```python
from build123d import *

# Parameters (mm, degrees)
BOSS_EXTRUDE1_DEPTH         = 4.7625
F_6_CLEARANCE_HOLE1_D       = 4.3053
F_3_4_0_75_DIAMETER_HOLE1_D = 19.05


with BuildPart() as part:
    # Sketch1 → Boss-Extrude1 (new body)
    with BuildSketch(Plane.XY):
        with BuildLine():
            Line((-159.14246691, -0.79375), (-164.887315329, -10.744119343))
            ThreePointArc((-164.887315329, -10.744119343), (-165.045907249, -11.126994109), (-165.1, -11.537869343))
            Line((-165.1, -11.537869343), (-165.1, -23.8125))
            ThreePointArc((-165.1, -23.8125), (-164.635032015, -24.935032015), (-163.5125, -25.4))
            Line((-163.5125, -25.4), (-1.5875, -25.4))
            ThreePointArc((-1.5875, -25.4), (-0.464967985, -24.935032015), (0, -23.8125))
            Line((0, -23.8125), (0, -1.5875))
            ThreePointArc((0, -1.5875), (-0.464967985, -0.464967985), (-1.5875, 0))
            Line((-1.5875, 0), (-157.767651581, 0))
            ThreePointArc((-157.767651581, 0), (-158.561401581, -0.212684671), (-159.14246691, -0.79375))
        make_face()
    extrude(amount=BOSS_EXTRUDE1_DEPTH)

    # #6 Clearance Hole1 (through all)
    with Locations(Plane.XY.offset(4.7625)):
        with Locations((-158.75, -18.415), (-117.475, -8.89), (-30.48, -16.51)):
            Hole(F_6_CLEARANCE_HOLE1_D / 2)

    # 3/4 (0.75) Diameter Hole1 (through all)
    with Locations(Plane.XY.offset(4.7625)):
        with Locations((-88.9, -10.16), (-53.975, -10.16), (-14.2875, -11.43)):
            Hole(F_3_4_0_75_DIAMETER_HOLE1_D / 2)


solid = part.part
```
Here's how the part is built. I have some questions about the finished solid (model axes, mm). Round coordinates to 2 decimals unless told otherwise and drop trailing zeros. Order: outer loops, then holes, each group sorted by start corner. A loop starts at its lowest first (then second) coordinate and runs counter-clockwise, first axis right, second up. Notation, with made-up numbers: (13, 76) -> (56, 76) arc R28 cw to (56, 111) -> close; hole circle Ø5 at (-5, 8). An arc over 180 degrees is marked (long way). Use a Markdown table: item, result. Add a question column.
(1) If we mould it in two halves opening along Y, with no side actions, what happens to faces 1 (the face through (-119.464, -9.714, 2.348)), 2 (the face through (-161.975, -5.699, 2.348)), 3 (the face through (-102, -13, 0))? For each: released by +Y, released by -Y, zero draft, split by the parting line, or undercut.
(2) I need wall thicknesses on line 1 along X through (y, z) = (-14, 2.85); line 2 along Y through (x, z) = (-30.48, 2.55); line 3 along Y through (x, z) = (-88.9, 2.1) (3 decimals). Which ranges of each line are inside material? Lowest first, please.
(3) Suppose I cut it at B-B, the plane z = 3.65. Count the separate pieces of the cut face and the enclosed holes in it, and give its area (3 significant figures).
(4) Suppose I cut it at A-A, the plane x = -30.48. Please give me the cut outline in (y, z), and give its area (3 significant figures).
Verdict:
| question | item | result |
|---|---|---|
| 1 | face 1 | undercut |
| 1 | face 2 | released by +Y |
| 1 | face 3 | zero draft |
| 2 | line 1 | -165.1 to -97.62, -80.18 to -62.69, -45.26 to -23.46, -5.12 to 0 |
| 2 | line 2 | -25.4 to -18.66, -14.36 to 0 |
| 2 | line 3 | -25.4 to -19.685, -0.635 to 0 |
| 3 | separate pieces | 1 |
| 3 | enclosed holes | 6 |
| 3 | area | 3,260 mm2 |
| 4 | outline | (-25.4, 0) -> (-18.66, 0) -> (-18.66, 4.76) -> (-25.4, 4.76) -> close; (-14.36, 0) -> (0, 0) -> (0, 4.76) -> (-14.36, 4.76) -> close |
| 4 | area | 100 mm2 |
